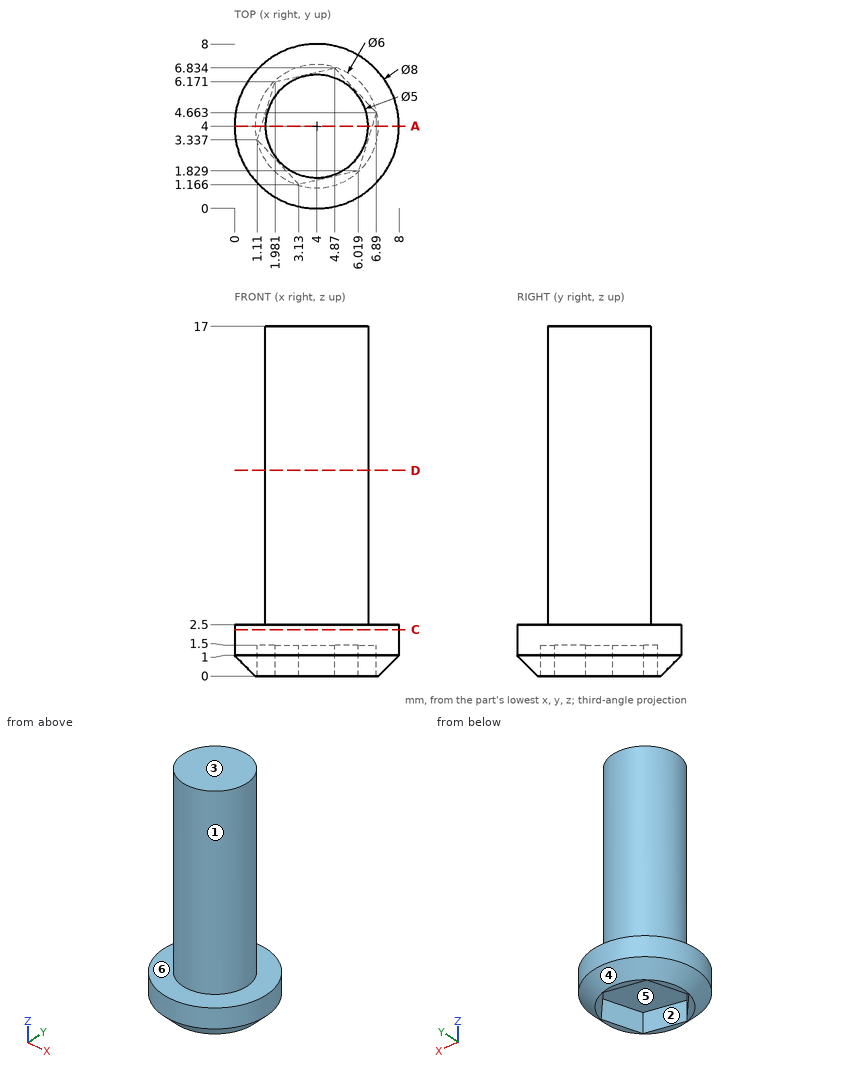
Here's the drawing with two shaded views (mm, measured from the low corner). I have some questions. A direction names the side the tool comes from. Give positions to 0.01 mm unless a question says otherwise; leave off trailing zeros. Order: outer loops, then holes, each group sorted by start corner. A loop starts at its lowest first (then second) coordinate and runs counter-clockwise, first axis right, second up.
Q1. For the marked faces 1, 2 and 3, which set-ups out of +Z, -Z, +X, -X, +Y, -Y let a thin tool reach every point of the face, with its end or its side?
Q2. I'm going to push flat-ended pins straight in: P1, Ø3, axis at y = 6.5, z = 8, coming from the +X side; P2, Ø1, axis at x = 1, y = 6.5, coming from the -Z side (1 decimal); P3, Ø2, axis at y = 7, z = 10, coming from the +X side. Where does each tip first touch, or does it pass through?
Q3. Suppose I cut it at A-A, the plane y = 4. Write out the boundary of the cut face in (x, z).
Q4. If I drill on line 1 along Z through (x, y) = (3.75, 5.25); line 2 along Y through (x, z) = (4, 7.5); line 3 along X through (y, z) = (4.25, 4.5), over which ranges is the centre line in solid material (lowest first)?
Q5. We'd pull the mould along X, two halves only. Please class the marked faces 4, 5 and 6: +X half, -X half, draft (parallel to the pull), parting line (faces both ways), or undercut.
Q6. Suppose I cut it at D-D, the plane z = 10. Write out the boundary of the cut face in (x, y).
Q7. Suppose I cut it at C-C, the plane z = 2.25. Write out the boundary of the cut face in (x, y).
Solution:
1. face 1: +Z
1. face 2: -Z
1. face 3: +Z, +X, -X, +Y, -Y
2. P1: stops at x = 6.29
2. P2: stops at z = 0.4
2. P3: stops at x = 5.5
3. outline: (0, 1) - (1, 0) - (1.31, 0) - (1.31, 1.5) - (6.69, 1.5) - (6.69, 0) - (7, 0) - (8, 1) - (8, 2.5) - (6.5, 2.5) - (6.5, 17) - (1.5, 17) - (1.5, 2.5) - (0, 2.5) - close
4. line 1: z = 1.5 to 17
4. line 2: y = 1.5 to 6.5
4. line 3: x = 1.51 to 6.49
5. face 4: parting line
5. face 5: undercut
5. face 6: draft
6. outline: circle Ø5 at (4, 4)
7. outline: circle Ø8 at (4, 4)
